For this review, take the finished solid that the model builds, in its own axes (mm). A direction names the side the tool comes from. Round coordinates to 2 decimals unless told otherwise and drop trailing zeros. Order: outer loops, then holes, each group sorted by start corner. A loop starts at its lowest first (then second) coordinate and runs counter-clockwise, first axis right, second up.
```python
from build123d import *

# Parameters (mm, degrees)
F1_DEPTH  = 30
F2_DEPTH  = 10
F0_W      = 250
F0_H      = 250
F0_H_2    = 30
F3_DEPTH  = 10
F6_DEPTH  = 250
F7_W      = 270
F7_H      = 270
F8_DEPTH  = 10
F9_DEPTH  = 20
F10_W     = 270
F10_H     = 5
F11_DEPTH = 330


with BuildPart() as f1:
    # F0 (on Top) → F1 (new body)
    with BuildSketch(Plane.XY):
        Polygon((125, -155), (155, -155), (155, 155), (-155, 155), (-155, -155), (-125, -155), (-125, -125), (-125, 125), (125, 125), (125, -125), align=None)
    extrude(amount=F1_DEPTH)

    # F0 (on Top) → F2 (join)
    with BuildSketch(Plane.XY):
        Polygon((155, -185), (155, -155), (125, -155), (-125, -155), (-155, -155), (-155, -185), align=None)
        Polygon((125, -155), (155, -155), (155, 155), (-155, 155), (-155, -155), (-125, -155), (-125, -125), (-125, 125), (125, 125), (125, -125), align=None)
    extrude(amount=F2_DEPTH)

    # F0 (on Top) → F3 (join)
    with BuildSketch(Plane.XY):
        Rectangle(F0_W, F0_H)
        Polygon((125, -155), (155, -155), (155, 155), (-155, 155), (-155, -155), (-125, -155), (-125, -125), (-125, 125), (125, 125), (125, -125), align=None)
        Polygon((155, -185), (155, -155), (125, -155), (-125, -155), (-155, -155), (-155, -185), align=None)
        with Locations((0, -140)):
            Rectangle(F0_W, F0_H_2)
    extrude(amount=F3_DEPTH)

    # F5 (on offset) → F6 (cut)
    with BuildSketch(Plane(origin=(-125, 0, 0), x_dir=(0, -1, 0), z_dir=(-1, 0, 0))):
        Polygon((155, 10), (185, 0), (185, 10), align=None)
    extrude(amount=-F6_DEPTH, mode=Mode.SUBTRACT)

    # F7 (on face) → F8 (cut)
    with BuildSketch(Plane(origin=(0, 0, 0), x_dir=(1, 0, 0), z_dir=(0, 0, -1))):
        Rectangle(F7_W, F7_H)
    extrude(amount=-F8_DEPTH, mode=Mode.SUBTRACT)

    # F9 (add): a face of the model
    f9_faces = [f1.faces().sort_by_distance(p)[0] for p in [
        (150.3989131719, -15, 0),
    ]]
    extrude(f9_faces, amount=F9_DEPTH)

    # F10 (on face) → F11 (cut)
    with BuildSketch(Plane.XZ.offset(185)):
        Polygon((145, -10), (-145, -10), (-145, -15), (-135, -15), (135, -15), (145, -15), align=None)
        with Locations((0, -17.5)):
            Rectangle(F10_W, F10_H)
    extrude(amount=-F11_DEPTH, mode=Mode.SUBTRACT)


solid = f1.part
```
Q1. Clearance check with flat-ended pins moving along their axes: pin 1 (3 mm diameter, centred on x = 84.5, y = -133, fed in from -Z) (1 decimal); pin 2 (3 mm diameter, centred on x = 21.5, z = -14.5, fed in from -Y); pin 3 (24 mm diameter, centred on x = -146.5, y = -175.5, fed in from +Z); pin 4 (1 mm diameter, centred on x = 78, z = 13, fed in from -Y). State where each tip first meets the part, or that it passes through.
Q2. Take a section at B-B, the plane x = -92. State the section outline as (y, z) points.
Q3. Mouldability with a two-part tool opening along X and no side actions: class faces 6 (the face through (-2, 145, -15)), 7 (the face through (-140, -155, 20)), 8 (the face through (-155, -17, 5)) as +X half, -X half, draft (parallel to the pull), parting line (faces both ways), or undercut.
Q4. Wall thickness on line 1 (Y direction, x = -5.5, z = -9.5); line 2 (X direction, y = -54.5, z = 1.5); line 3 (X direction, y = -112, z = 26): over which ranges is each line inside the solid? List them lowest first.
Q5. Take a section at A-A, the plane y = 11. State the section outline as (x, z) points, plus the area to 3 significant figures.
Q6. Tool access review of faces 1 (the face through (-140, -170, 10)), 2 (the face through (140, -22, -15)), 3 (the face through (-2, 125, 20)), 4 (the face through (-2, -170, 5)), 5 (the face through (-2, 135, 0)): name each direction out of +Z, -Z, +X, -X, +Y, -Y from which nothing blocks a thin tool from reaching the whole face with its end or side.
Q7. Take a section at C-C, the plane z = 24. State the section outline as (x, y) points, plus the area to 3 significant figures.
Working result:
1. pin 1: passes through
1. pin 2: stops at y = 145
1. pin 3: stops at z = 10
1. pin 4: stops at y = 125
2. outline: (-185, -10) - (-135, -10) - (-135, 10) - (-155, 10) - (-185, 0) - close; (125, 10) - (135, 10) - (135, -10) - (145, -10) - (145, -20) - (155, -20) - (155, 30) - (125, 30) - close
3. face 6: undercut
3. face 7: draft
3. face 8: -X half
4. line 1: y = -185 to -135, 135 to 155
4. line 2: x = -155 to -135, 135 to 155
4. line 3: x = -155 to -125, 125 to 155
5. outline: (-155, -20) - (-135, -20) - (-135, -15) - (-145, -15) - (-145, -10) - (-135, -10) - (-135, 10) - (-125, 10) - (-125, 30) - (-155, 30) - close; (125, 10) - (135, 10) - (135, -10) - (145, -10) - (145, -15) - (135, -15) - (135, -20) - (155, -20) - (155, 30) - (125, 30) - close
5. area: 2,300 mm2
6. face 1: +Z, +X, -X, -Y
6. face 2: -Y
6. face 3: +Z, -Z, -Y
6. face 4: +Z, -Y
6. face 5: -Z
7. outline: (-155, -155) - (-125, -155) - (-125, 125) - (125, 125) - (125, -155) - (155, -155) - (155, 155) - (-155, 155) - close
7. area: 26,100 mm2
